Model file for the job. Use its own axes, mm. Coordinates: 2 decimals unless noted, no trailing zeros. Order: outer loops, then holes, each group sorted by start corner. A loop starts at its lowest first (then second) coordinate and runs counter-clockwise, first axis right, second up. Notation, with made-up numbers: M 76,-35 L 117,-35 A6 cw 117,-29 Z; hole C -24,23.25 d9. An arc over 180 degrees is marked long. Return JSON: item names as keys, results as strings.
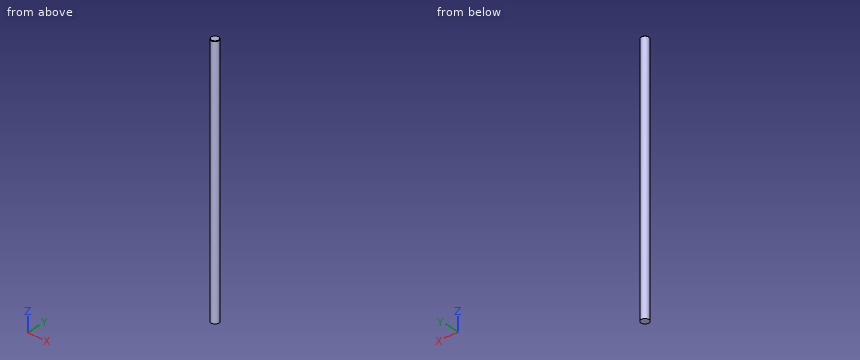
```python
from build123d import *

# Parameters (mm, degrees)
SKETCH3_R           = 3
BOSS_EXTRUDE1_DEPTH = 152.4
CHAMFER1_SIZE       = 0.375
SKETCH4_R           = 3
CUT_EXTRUDE1_DEPTH  = 191.047362518


with BuildPart() as part:
    # Sketch3 → Boss-Extrude1 (new, symmetric)
    with BuildSketch(Plane.XY):
        with Locations(Location((0, 0, 0), (0, 0, 180))):
            Circle(SKETCH3_R)
    extrude(amount=BOSS_EXTRUDE1_DEPTH, both=True)

    # Chamfer1
    chamfer1_edges = [part.edges().sort_by_distance(p)[0] for p in [
        (3, 0, -152.4),
        (3, 0, 152.4),
    ]]
    chamfer(chamfer1_edges, length=CHAMFER1_SIZE)

    # Sketch4 → Cut-Extrude1 (cut, through all)
    with BuildSketch(Plane.XY.offset(-37.6)):
        with Locations(Location((0, 0, 0), (0, 0, 180))):
            Circle(SKETCH4_R)
    extrude(amount=-CUT_EXTRUDE1_DEPTH, mode=Mode.SUBTRACT)


solid = part.part
```
Item 1: Saw through at A-A (z = 69.5). Write the cut outline in (x, y).
Check result:
{"outline": "C 0,0 d6"}
Item 2: Drop a flat-ended pin along its axis: pin 1 Ø1 at (y, z) = (-1, 129) entering from -X. Give the stop position or say it passes through.
Check result:
{"pin 1": "stops at x = -2.96"}
Item 3: Wall check: line 1 (X direction, y = -0.1, z = 105); line 2 (X direction, y = -1.4, z = 15.5). Give the ranges that are in metal, low to high.
Check result:
{"line 1": "x = -3 to 3", "line 2": "x = -2.65 to 2.65"}
